Can you work these out from the drawing? Everything is in mm from the part's minimum corner. A direction names the side the tool comes from. Coordinates: 2 decimals unless noted, no trailing zeros. Write each loop counter-clockwise with the first axis right and the second up, starting at its lowest first coordinate (ties: lowest second). Pieces come first, ordered by that corner, then holes. Notation, with made-up numbers: (52, 4) -> (109, 4) arc R17 cw to (109, 15) -> close; hole circle Ø10 at (-29.75, 84). An arc over 180 degrees is marked (long way). Use a Markdown table: item, result. Add a question column.
Item 1: Imagine slicing it at A-A, the plane z = 2. Write out the boundary of the cut face in (x, y).
Item 2: If I drill on line 1 along Z through (x, y) = (27, 7); line 2 along X through (y, z) = (2.25, 3.5); line 3 along Z through (x, y) = (27.5, 11.5), over which ranges is the centre line in solid material (lowest first)? Write a range as from..to.
Item 3: Will these pins go through, and if not, where does the flat tip stop? pin 1 Ø3.5 at (x, y) = (31.5, 8.5) entering from -Z; pin 2 Ø10 at (x, y) = (31, 9) entering from +Z; pin 3 Ø4 at (x, y) = (31, 5) entering from +Z.
Item 4: Imagine slicing it at D-D, the plane z = 6.75. Write out the boundary of the cut face in (x, y) (3 decimals), and give its area (3 significant figures).
Item 5: Imagine slicing it at C-C, the plane x = 34.5. Write out the boundary of the cut face in (y, z) (3 decimals), and give its area (3 significant figures).
Item 6: Imagine slicing it at B-B, the plane y = 10.5. Write out the boundary of the cut face in (x, z), and give its area (3 significant figures).
Item 7: On a 3-axis mill with a long thin cutter (end or side, diameter ignored), from which of +Z, -Z, +X, -X, +Y, -Y can I reach the whole of each face in a straight line? I mean the marked faces 1, 2, 3 and 4. Say none if no direction works.
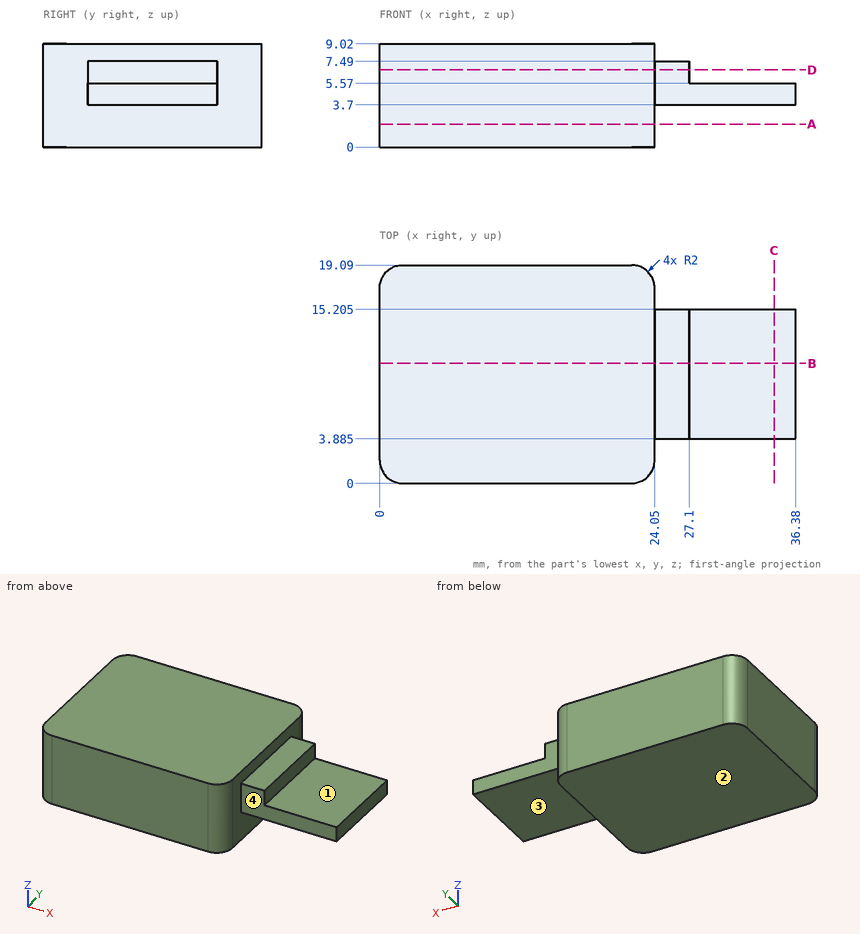
Ans:
| question | item | result |
|---|---|---|
| 1 | outline | (0, 2) arc R2 ccw to (2, 0) -> (22.05, 0) arc R2 ccw to (24.05, 2) -> (24.05, 17.09) arc R2 ccw to (22.05, 19.09) -> (2, 19.09) arc R2 ccw to (0, 17.09) -> close |
| 2 | line 1 | z = 3.7..7.49 |
| 2 | line 2 | x = 0..24.05 |
| 2 | line 3 | z = 3.7..5.57 |
| 3 | pin 1 | stops at z = 3.7 |
| 3 | pin 2 | stops at z = 7.49 |
| 3 | pin 3 | stops at z = 5.57 |
| 4 | outline | (0, 2) arc R2 ccw to (2, 0) -> (22.05, 0) arc R2 ccw to (24.05, 2) -> (24.05, 3.885) -> (27.1, 3.885) -> (27.1, 15.205) -> (24.05, 15.205) -> (24.05, 17.09) arc R2 ccw to (22.05, 19.09) -> (2, 19.09) arc R2 ccw to (0, 17.09) -> close |
| 4 | area | 490 mm^2 |
| 5 | outline | (3.885, 3.7) -> (15.205, 3.7) -> (15.205, 5.57) -> (3.885, 5.57) -> close |
| 5 | area | 21.2 mm^2 |
| 6 | outline | (0, 0) -> (24.05, 0) -> (24.05, 3.7) -> (36.38, 3.7) -> (36.38, 5.57) -> (27.1, 5.57) -> (27.1, 7.49) -> (24.05, 7.49) -> (24.05, 9.02) -> (0, 9.02) -> close |
| 6 | area | 246 mm^2 |
| 7 | face 1 | +Z, +X, +Y, -Y |
| 7 | face 2 | -Z, +X, -X, +Y, -Y |
| 7 | face 3 | -Z, +X, +Y, -Y |
| 7 | face 4 | +Z, -Z, +X, -Y |
